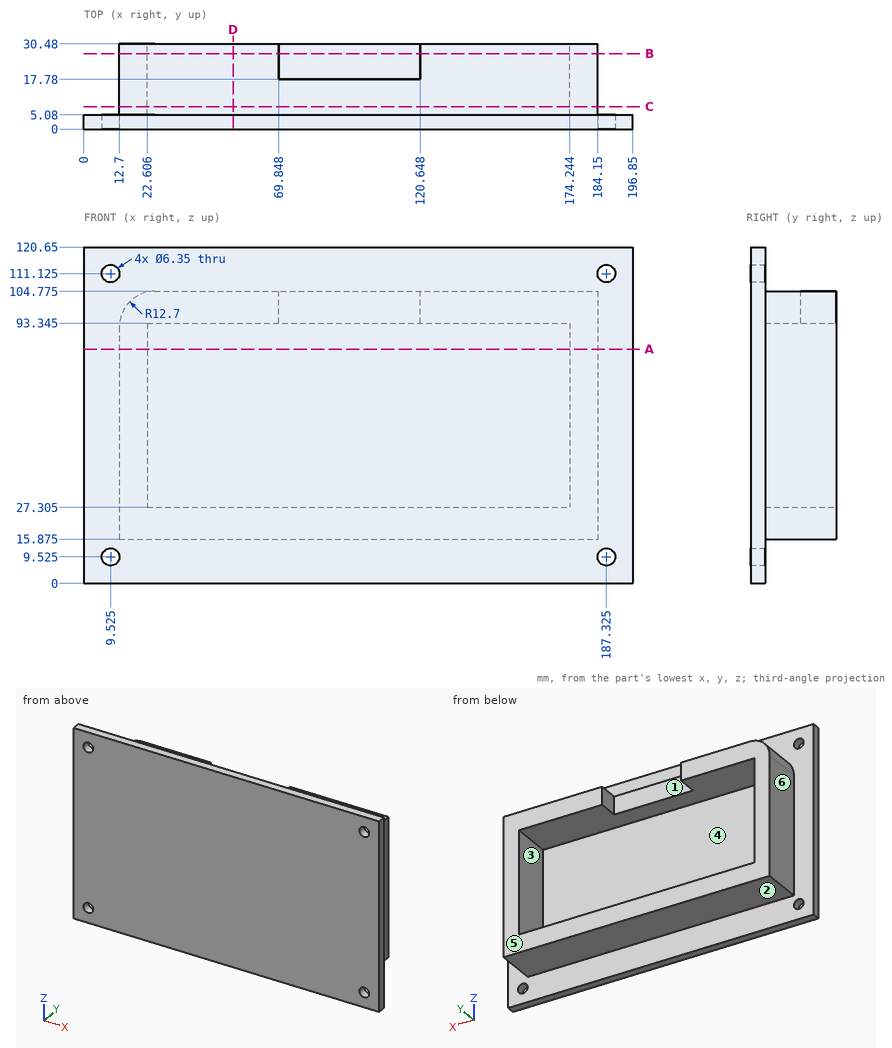
For this review, use the dimensioned drawing (mm, ordinates from the lowest corner) and the shaded views. A direction names the side the tool comes from. Give positions to 0.01 mm unless a question says otherwise; leave off trailing zeros. Write each loop counter-clockwise with the first axis right and the second up, starting at its lowest first coordinate (ties: lowest second). Pieces come first, ordered by that corner, then holes. Notation, with made-up numbers: M 25.5,3 L 76.5,3 A32 cw 76.5,37 Z; hole C -6,24 d10. An arc over 180 degrees is marked long. Write item = value, one per line. Start each with the question number.
Q1. Machinability: for the marked faces 1, 2 and 3, which of the approach directions +Z, -Z, +X, -X, +Y, -Y give a long, thin tool a straight path to every point of the face, cutting with its end or side? Answer none if there is none.
Q2. We need section A-A (z = 84). State the section outline as (x, y) points, plus the area to 3 significant figures.
Q3. Mouldability with a two-part tool opening along X and no side actions: class the marked faces 4, 5 and 6 as released by +X, released by -X, zero draft, split by the parting line, or undercut.
Q4. Clearance check with flat-ended pins moving along their axes: pin 1 (12.5 mm diameter, centred on y = 27, z = 101.5, fed in from +X); pin 2 (8 mm diameter, centred on x = 131, y = 21, fed in from +Z) (3 decimals); pin 3 (9 mm diameter, centred on y = 21, z = 101.5, fed in from -X); pin 4 (8.5 mm diameter, centred on x = 187.325, z = 9.525, fed in from -Y). State where each tip first meets the part, or that it passes through.
Q5. We need section D-D (x = 53.5). State the section outline as (y, z) points (3 decimals), plus the area to 3 significant figures.
Q6. We need section B-B (y = 27). State the section outline as (x, z) points (3 decimals), plus the area to 3 significant figures.
Q7. For line 1 (X direction, y = 29, z = 61); line 2 (Z direction, x = 47.5, y = 11) (3 decimals); line 3 (X direction, y = 4, z = 111), list the stretches that pass through material, from the lowest coordinate up.
Q8. We need section C-C (y = 8). State the section outline as (x, z) points (3 decimals), plus the area to 3 significant figures.
Result set:
q1.face_1 = +Z, +Y
q1.face_2 = -Z, +X, -X, +Y
q1.face_3 = +Y
q2.outline = M 0,0 L 196.85,0 L 196.85,5.08 L 184.15,5.08 L 184.15,30.48 L 174.24,30.48 L 174.24,5.08 L 22.61,5.08 L 22.61,30.48 L 12.7,30.48 L 12.7,5.08 L 0,5.08 Z
q2.area = 1,500 mm2
q3.face_4 = undercut
q3.face_5 = zero draft
q3.face_6 = released by -X
q4.pin_1 = 184.15
q4.pin_2 = 104.775
q4.pin_3 = 13.69
q4.pin_4 = 0
q5.outline = M 0,0 L 5.08,0 L 5.08,15.875 L 30.48,15.875 L 30.48,27.305 L 5.08,27.305 L 5.08,93.345 L 30.48,93.345 L 30.48,104.775 L 5.08,104.775 L 5.08,120.65 L 0,120.65 Z
q5.area = 1,190 mm2
q6.outline = M 12.7,15.875 L 184.15,15.875 L 184.15,104.775 L 120.648,104.775 L 120.648,93.345 L 174.244,93.345 L 174.244,27.305 L 22.606,27.305 L 22.606,93.345 L 69.848,93.345 L 69.848,104.775 L 25.4,104.775 A12.7 ccw 12.7,92.075 Z
q6.area = 4,610 mm2
q7.line_1 = 12.7 to 22.61, 174.24 to 184.15
q7.line_2 = 15.875 to 27.305, 93.345 to 104.775
q7.line_3 = 0 to 6.35, 12.7 to 184.15, 190.5 to 196.85
q8.outline = M 12.7,15.875 L 184.15,15.875 L 184.15,104.775 L 25.4,104.775 A12.7 ccw 12.7,92.075 Z; hole M 22.606,27.305 L 174.244,27.305 L 174.244,93.345 L 22.606,93.345 Z
q8.area = 5,190 mm2
